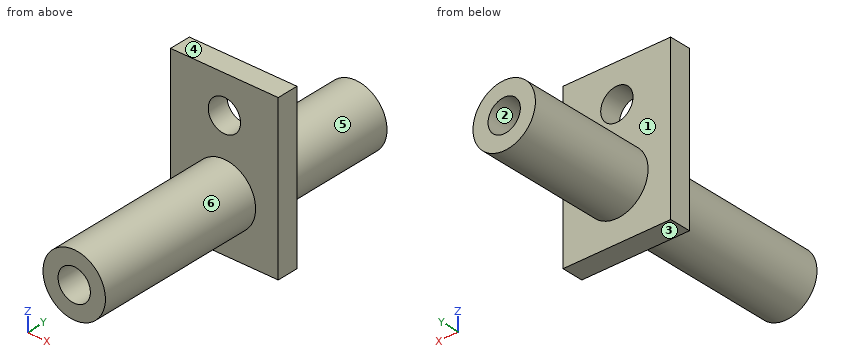
from build123d import *

# Parameters (mm, degrees)
SKETCH_1_R          = 2.9
SKETCH_1_R_2        = 1.5
EXTRUDE_1_DEPTH     = 40
SKETCH_2_W          = 10
SKETCH_2_H          = 15
SKETCH_2_R          = 1.5
EXTRUDE_2_DEPTH     = 2
SKETCH_3_R          = 2.9
CUT_EXTRUDE_1_DEPTH = 33.015621187


with BuildPart() as part:
    # 草图1 → 凸台-拉伸1 (new body)
    with BuildSketch(Plane(origin=(0, 0, 0), x_dir=(1, 0, 0), z_dir=(0, 1, 0))):
        with Locations(Location((0, 0, 0), (0, 0, 270))):
            Circle(SKETCH_1_R)
        with Locations(Location((0, 0, 0), (0, 0, 270))):
            Circle(SKETCH_1_R_2, mode=Mode.SUBTRACT)
    extrude(amount=EXTRUDE_1_DEPTH)

    # 草图2 → 凸台-拉伸2 (add)
    with BuildSketch(Plane(origin=(0, 28, 0), x_dir=(1, 0, 0), z_dir=(0, 1, 0))):
        with Locations((0, -2.5)):
            Rectangle(SKETCH_2_W, SKETCH_2_H)
        with Locations(Location((0, -6.5, 0), (0, 0, 270))):
            Circle(SKETCH_2_R, mode=Mode.SUBTRACT)
    extrude(amount=-EXTRUDE_2_DEPTH)

    # 草图3 → 切除-拉伸1 (cut, through all)
    with BuildSketch(Plane(origin=(0, 10, 0), x_dir=(-1, 0, 0), z_dir=(0, -1, 0))):
        with Locations(Location((0, 0, 0), (0, 0, 90))):
            Circle(SKETCH_3_R)
    extrude(amount=CUT_EXTRUDE_1_DEPTH, mode=Mode.SUBTRACT)


solid = part.part
The model under review builds one solid part; all positions refer to its coordinate system, in mm. Face numbers are marked on the shaded views. A direction names the side the tool comes from. Coordinates: 2 decimals unless noted, no trailing zeros. Order: outer loops, then holes, each group sorted by start corner. A loop starts at its lowest first (then second) coordinate and runs counter-clockwise, first axis right, second up. Notation, with made-up numbers: (55, -1.75) -> (84, -1.75) arc R22 cw to (84, 29.25) -> close; hole circle Ø9 at (87, 40). An arc over 180 degrees is marked (long way). Answer in a Markdown table with one row per item.
(1) Consider section D-D (z = -4). Write out the cut boundary in (x, y).
Answers:
| item | result |
|---|---|
| outline | (-5, 26) -> (5, 26) -> (5, 28) -> (-5, 28) -> close |
(2) Consider section B-B (z = 6.5). Write out the cut boundary in (x, y).
Answers:
| item | result |
|---|---|
| outline | (-5, 26) -> (-1.5, 26) -> (-1.5, 28) -> (-5, 28) -> close; (1.5, 26) -> (5, 26) -> (5, 28) -> (1.5, 28) -> close |
(3) The part is to be moulded in two halves that separate along Z. For the marked faces 1, 2 and 3, say which applies: +Z half, -Z half, draft (parallel to the pull), parting line (faces both ways), or undercut.
Answers:
| item | result |
|---|---|
| face 1 | draft |
| face 2 | undercut |
| face 3 | -Z half |
(4) Consider section A-A (x = 0). Write out the cut boundary in (y, z).
Answers:
| item | result |
|---|---|
| outline | (10, -2.9) -> (26, -2.9) -> (26, -5) -> (28, -5) -> (28, -2.9) -> (40, -2.9) -> (40, -1.5) -> (28, -1.5) -> (28, 1.5) -> (40, 1.5) -> (40, 2.9) -> (28, 2.9) -> (28, 5) -> (26, 5) -> (26, 2.9) -> (10, 2.9) -> (10, 1.5) -> (26, 1.5) -> (26, -1.5) -> (10, -1.5) -> close; (26, 8) -> (28, 8) -> (28, 10) -> (26, 10) -> close |
(5) Consider section C-C (y = 37). Write out the cut boundary in (x, z), plus the area to 3 significant figures.
Answers:
| item | result |
|---|---|
| outline | circle Ø5.8 at (0, 0); hole circle Ø3 at (0, 0) |
| area | 19.4 mm² |
(6) Machinability: for the marked faces 4, 5 and 6, which of the approach directions +Z, -Z, +X, -X, +Y, -Y give a long, thin tool a straight path to every point of the face, cutting with its end or side? Answer none if there is none.
Answers:
| item | result |
|---|---|
| face 4 | +Z, +X, -X, +Y, -Y |
| face 5 | +Y |
| face 6 | -Y |
(7) Insertion check: pin 1 (1 mm diameter, centred on x = -1.5, z = 5, fed in from +Y); pin 2 (0.9 mm diameter, centred on x = -0.5, z = 0.5, fed in from -Y); pin 3 (8 mm diameter, centred on y = 18.5, z = 5.5, fed in from -X). Each pin has a flat end and moves straight along its axis. Give the tip position at first contact, or say it passes through.
Answers:
| item | result |
|---|---|
| pin 1 | y = 28 |
| pin 2 | y = 26 |
| pin 3 | x = -2.48 |
(8) Wall thickness on line 1 along Z through (x, y) = (0, 37.5); line 2 along Y through (x, z) = (2, 4.5): over which ranges is each line inside the solid? List them lowest first.
Answers:
| item | result |
|---|---|
| line 1 | -2.9 to -1.5, 1.5 to 2.9 |
| line 2 | 26 to 28 |
